Part model, mm, in its own coordinate system. Face numbers are marked on the shaded views. A direction names the side the tool comes from. Coordinates: 2 decimals unless noted, no trailing zeros. Write each loop counter-clockwise with the first axis right and the second up, starting at its lowest first coordinate (ties: lowest second). Pieces come first, ordered by that corner, then holes. Notation, with made-up numbers: (66, 5.5) -> (114, 5.5) arc R19 cw to (114, 18.5) -> close; hole circle Ø1 at (78.5, 25). An arc over 180 degrees is marked (long way). Write item = value, one per line.
from build123d import *

# Parameters (mm, degrees)
SKETCH_1_R          = 12.5
EXTRUDE_1_DEPTH     = 8
EXTRUDE_START       = -8
SKETCH_2_R          = 12.5
EXTRUDE_2_DEPTH     = 8
CUT_EXTRUDE_6_DEPTH = 30
EXTRUDE_START_2     = -0.031547984
EXTRUDE_3_DEPTH     = 4.031547984
MIRROR_START        = -16
MIRROR_1_OUTLINE_R  = 12.5
MIRROR_1_DEPTH      = 8
MIRROR_START_2      = -8.031547984
MIRROR_1_2_DEPTH    = 4.031547984


# Read off the part's stored shape, not the designer's step: 镜向1
with BuildPart() as part:
    # 草图1 → 凸台-拉伸1 (new body)
    with BuildSketch(Plane.XY):
        with BuildLine():
            Line((-49.218570577, 33.143230451), (-9.339427202, -11.685933312))
            ThreePointArc((-9.339427202, -11.685933312), (-10.860056091, -37.708027961), (-36.882150741, -36.187399071))
            Line((-36.882150741, -36.187399071), (-76.761294116, 8.641764691))
            ThreePointArc((-76.761294116, 8.641764691), (-75.240665226, 34.663859341), (-49.218570577, 33.143230451))
        make_face()
        with Locations((-23.110788971, -23.936666192)):
            Circle(SKETCH_1_R, mode=Mode.SUBTRACT)
        with Locations((-62.989932346, 20.892497571)):
            Circle(SKETCH_1_R, mode=Mode.SUBTRACT)
    extrude(amount=EXTRUDE_1_DEPTH)

    # 草图2 → 凸台-拉伸2 (add)
    with BuildSketch(Plane.XY.offset(8).offset(EXTRUDE_START)):
        with BuildLine():
            Line((-81.224750465, 18.616304916), (-93.707423119, 118.616304916))
            ThreePointArc((-93.707423119, 118.616304916), (-77.748797655, 139.12731569), (-57.237786881, 123.168690226))
            Line((-57.237786881, 123.168690226), (-44.755114228, 23.168690226))
            ThreePointArc((-44.755114228, 23.168690226), (-60.713739692, 2.657679452), (-81.224750465, 18.616304916))
        make_face()
        with Locations((-62.989932346, 20.892497571)):
            Circle(SKETCH_2_R, mode=Mode.SUBTRACT)
        with Locations((-75.472605, 120.892497571)):
            Circle(SKETCH_2_R, mode=Mode.SUBTRACT)
    extrude(amount=EXTRUDE_2_DEPTH)

    # 草图4 → 切除-拉伸6 (cut)
    with BuildSketch(Plane.XY.offset(8)):
        with BuildLine():
            Line((-50.286228122, 27.138087208), (-32.136603064, 6.778447679))
            ThreePointArc((-32.136603064, 6.778447679), (-33.211064798, -11.943932547), (-51.933445024, -10.869470813))
            Line((-51.933445024, -10.869470813), (-72.45355192, 12.149295588))
            ThreePointArc((-72.45355192, 12.149295588), (-75.02839357, 16.472286713), (-75.807301146, 21.443339396))
            Line((-75.807301146, 21.443339396), (-83.815726922, 75.482800481))
            ThreePointArc((-83.815726922, 75.482800481), (-72.828124355, 90.29362358), (-58.017301256, 79.306021012))
            Line((-58.017301256, 79.306021012), (-50.286228122, 27.138087208))
        make_face()
    extrude(amount=-CUT_EXTRUDE_6_DEPTH, mode=Mode.SUBTRACT)

    # 草图5 → 凸台-拉伸3 (add)
    with BuildSketch(Plane(origin=(0, 0, 0), x_dir=(-1, 0, 0), z_dir=(0, 0, -1)).offset(EXTRUDE_START_2)):
        Polygon((48.100432454, 49.968385441), (84.570068691, 45.416000132), (81.591125202, 21.551371363), (80.712358407, 15.828262623), (79.125142105, 11.982622874), (76.761294116, 8.641764691), (63.001048061, -6.826479398), (33.316578165, 15.267394572), (45.474886231, 28.934859247), align=None)
    extrude(amount=EXTRUDE_3_DEPTH)



with BuildPart() as body_2:
    # 镜向1 outline → 镜向1 (new body)
    with BuildSketch(Plane.XY.offset(MIRROR_START)):
        with BuildLine():
            ThreePointArc((-81.401718429, 20.034013842), (-80.059923167, 13.939349041), (-76.761294116, 8.641764691))
            Line((-76.761294116, 8.641764691), (-36.882150741, -36.187399071))
            ThreePointArc((-36.882150741, -36.187399071), (-10.860056092, -37.708027961), (-9.339427202, -11.685933312))
            Line((-9.339427202, -11.685933312), (-45.474886231, 28.934859247))
            Line((-45.474886231, 28.934859247), (-57.237786881, 123.168690226))
            ThreePointArc((-57.237786881, 123.168690226), (-77.748797655, 139.12731569), (-93.707423119, 118.616304916))
            Line((-93.707423119, 118.616304916), (-81.401718429, 20.034013842))
        make_face()
        with BuildLine():
            Line((-75.807301146, 21.443339396), (-83.815726922, 75.482800481))
            ThreePointArc((-83.815726922, 75.482800481), (-72.828124355, 90.29362358), (-58.017301256, 79.306021012))
            Line((-58.017301256, 79.306021012), (-50.286228122, 27.138087208))
            Line((-50.286228122, 27.138087208), (-32.136603064, 6.778447679))
            ThreePointArc((-32.136603064, 6.778447679), (-33.211064798, -11.943932547), (-51.933445024, -10.869470813))
            Line((-51.933445024, -10.869470813), (-72.45355192, 12.149295588))
            ThreePointArc((-72.45355192, 12.149295588), (-75.02839357, 16.472286713), (-75.807301146, 21.443339396))
        make_face(mode=Mode.SUBTRACT)
        with Locations((-75.472605, 120.892497571)):
            Circle(MIRROR_1_OUTLINE_R, mode=Mode.SUBTRACT)
        with Locations((-23.110788971, -23.936666192)):
            Circle(MIRROR_1_OUTLINE_R, mode=Mode.SUBTRACT)
    extrude(amount=MIRROR_1_DEPTH)


with BuildPart() as part_1:
    add(part.part)

    add(body_2.part)  # Mirror 1 2 merges body 2
    # Mirror 1 2 outline → Mirror 1 2 (add)
    with BuildSketch(Plane.XY.offset(MIRROR_START_2)):
        Polygon((-81.591125202, 21.551371363), (-80.712358407, 15.828262623), (-79.125142105, 11.982622874), (-76.761294116, 8.641764691), (-63.001048061, -6.826479398), (-33.316578165, 15.267394572), (-45.474886231, 28.934859247), (-48.100432453, 49.968385441), (-84.570068691, 45.416000132), align=None)
    extrude(amount=MIRROR_1_2_DEPTH)


solid = part_1.part
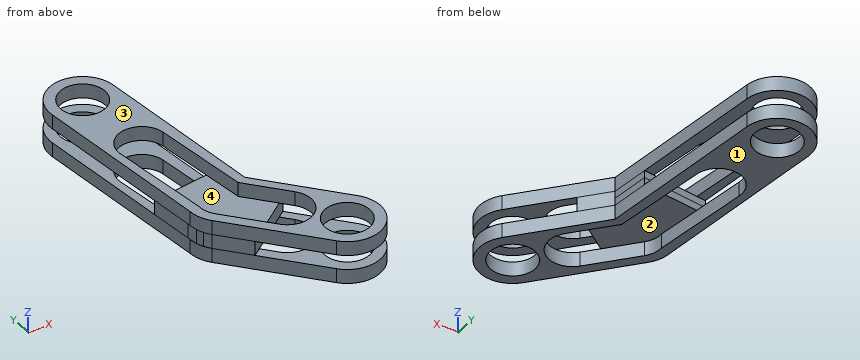
Q1. Saw through at D-D on y = 99.5. Give the cut face in (x, z), and give its area (3 significant figures).
Model answer:
outline = (-91.32, -16) -> (-54.28, -16) -> (-54.28, -8) -> (-91.32, -8) -> close; (-91.32, 0) -> (-54.28, 0) -> (-54.28, 8) -> (-91.32, 8) -> close
area = 593 mm²
Q2. Pin check, flat tips, straight feed: pin 1 (6 mm diameter, centred on y = 50, z = 4.5, fed in from +X); pin 2 (0.8 mm diameter, centred on x = -80, y = 13, fed in from +Z); pin 3 (4 mm diameter, centred on y = 83.5, z = -11, fed in from -X); pin 4 (10 mm diameter, centred on x = -83, z = -5, fed in from +Y). Stop position of each tip, or through.
Model answer:
pin_1 = -47.73
pin_2 = 8
pin_3 = -89.57
pin_4 = 138.93
Q3. Saw through at B-B on x = -15.5. Give the cut face in (y, z).
Model answer:
outline = (-40.72, -16) -> (-33.85, -16) -> (-33.85, -8) -> (-40.72, -8) -> close; (-40.72, 0) -> (-33.85, 0) -> (-33.85, 8) -> (-40.72, 8) -> close; (-14.02, -16) -> (-4.76, -16) -> (-4.76, -8) -> (-14.02, -8) -> close; (-14.02, 0) -> (-4.76, 0) -> (-4.76, 8) -> (-14.02, 8) -> close
Q4. Probe line 1 (Z direction, x = -85.5, y = 71.5); line 2 (Y direction, x = -13, z = 4.5); line 3 (Y direction, x = -30.5, z = 2.5). List the from-to ranges inside material, lowest first. Write a range as from..to.
Model answer:
line_1 = -16..-8, 0..8
line_2 = -39.35..-31.29, -16.59..-7.57
line_3 = -40.82..-34.02, -13.85..-8.59, 4.5..12.1
Q5. Which spindle directions (+Z, -Z, +X, -X, +Y, -Y) get a long thin tool onto all of the face, cutting with end or side? Do the marked faces 3 and 4. Say none if no direction does.
Model answer:
face_3 = +Z, +X, -X, +Y, -Y
face_4 = +Z
Q6. Saw through at A-A on y = 127. Give the cut face in (x, z).
Model answer:
outline = (-92.8, -16) -> (-86.38, -16) -> (-86.38, -8) -> (-92.8, -8) -> close; (-92.8, 0) -> (-86.38, 0) -> (-86.38, 8) -> (-92.8, 8) -> close; (-64.57, -16) -> (-58.14, -16) -> (-58.14, -8) -> (-64.57, -8) -> close; (-64.57, 0) -> (-58.14, 0) -> (-58.14, 8) -> (-64.57, 8) -> close
Q7. Mould opens along X. For the marked faces 1 and 2 say: released by +X, released by -X, zero draft, split by the parting line, or undercut.
Model answer:
face_1 = zero draft
face_2 = undercut
Q8. Saw through at C-C on x = -60.5. Give the cut face in (y, z), and give its area (3 significant figures).
Model answer:
outline = (-9.64, -16) -> (-1.26, -16) -> (-1.26, -8.03) -> (48.42, -8.03) -> (48.42, 0.03) -> (-1.26, 0.03) -> (-1.26, 8) -> (-9.64, 8) -> (-9.64, 0) -> (-4.96, 0) -> (-4.96, -8) -> (-9.64, -8) -> close; (85.24, -16) -> (131.55, -16) -> (131.55, -8) -> (85.24, -8) -> close; (85.24, 0) -> (131.55, 0) -> (131.55, 8) -> (85.24, 8) -> close
area = 1,310 mm²
